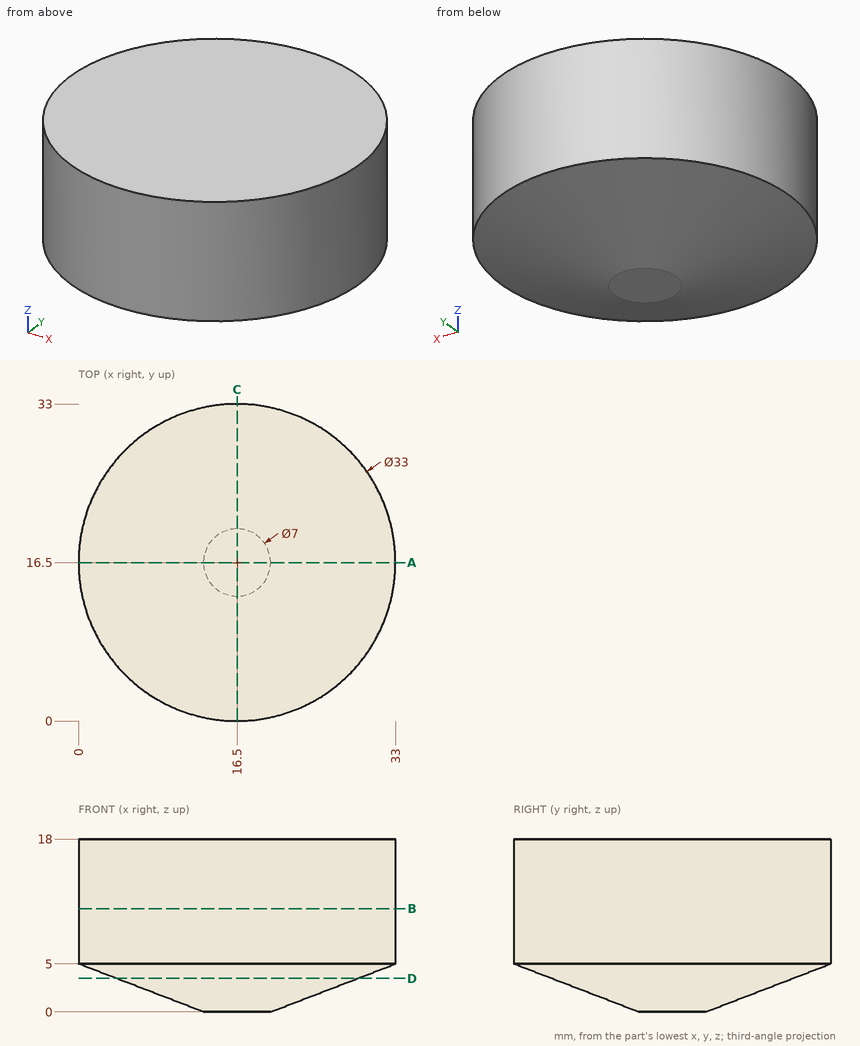
For this review, use the dimensioned drawing (mm, ordinates from the lowest corner) and the shaded views. Coordinates: 2 decimals unless noted, no trailing zeros. Order: outer loops, then holes, each group sorted by start corner. A loop starts at its lowest first (then second) coordinate and runs counter-clockwise, first axis right, second up. Notation, with made-up numbers: (-26, 88) - (-1, 88) arc R27 ccw to (-1, 107) - close; hole circle Ø4 at (-1.5, 59.5). An arc over 180 degrees is marked (long way). Use one line per item in the form item = value.
Q1. For P1, Ø10, axis at x = 25.5, z = 4, coming from the +Y side; P2, Ø1.5, axis at x = 23.5, z = 11, coming from the -Y side; P3, Ø3, axis at y = 7, z = 15, coming from the +X side, all flat-tipped, find the tip position at first contact; note any pin that passes through.
Checked values:
P1 = 32.48
P2 = 1.23
P3 = 30.93
Q2. Consider section B-B (z = 10.75). Give the boundary of the cut face in (x, y), then the cut area to 3 significant figures.
Checked values:
outline = circle Ø33 at (16.5, 16.5)
area = 855 mm2
Q3. Consider section A-A (y = 16.5). Give the boundary of the cut face in (x, z), then the cut area to 3 significant figures.
Checked values:
outline = (0, 5) - (13, 0) - (20, 0) - (33, 5) - (33, 18) - (0, 18) - close
area = 529 mm2
Q4. Consider section D-D (z = 3.5). Give the boundary of the cut face in (x, y), then the cut area to 3 significant figures.
Checked values:
outline = circle Ø25.2 at (16.5, 16.5)
area = 499 mm2
Q5. For probe 1 along Y at (x, z) = (27.5, 17); probe 2 along Z at (x, y) = (16.5, 12.5); probe 3 along Y at (x, z) = (16, 6), list the stretches that pass through material, from the lowest coordinate up. Write a range as from..to.
Checked values:
probe_1 = 4.2..28.8
probe_2 = 0.19..18
probe_3 = 0.01..32.99
